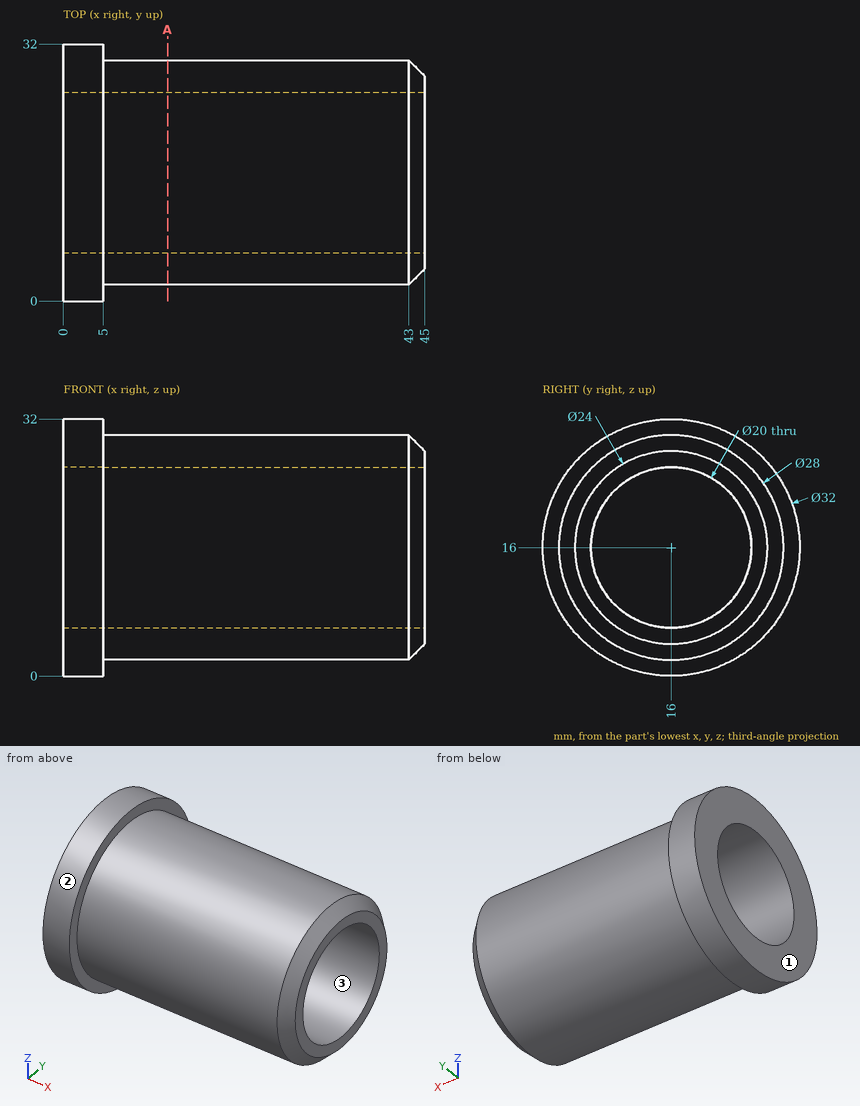
Could you check a few things on this drawing? It's one solid part, dimensions in mm from its lowest x, y, z. Give positions to 0.01 mm unless a question says otherwise; leave off trailing zeros. Order: outer loops, then holes, each group sorted by start corner. A loop starts at its lowest first (then second) coordinate and runs counter-clockwise, first axis right, second up. Notation, with made-up numbers: (20, 71.25) - (62, 71.25) arc R37 ccw to (62, 108.25) - close; hole circle Ø11 at (69, 43). An arc over 180 degrees is marked (long way). One line per item, written item: value. Start each with the question number.
1. Imagine slicing it at A-A on x = 13. List the corners of the cut face in (y, z) for me.
2. Thinking about a two-plate mould opening in Z: for the marked faces 1, 2 and 3, which applies, +Z half, -Z half, draft (parallel to the pull), parting line (faces both ways), or undercut?
3. For P1, Ø10, axis at x = 27, z = 20, coming from the +Y side; P2, Ø8, axis at x = 30, y = 6.5, coming from the -Z side; P3, Ø6, axis at x = 35, y = 24, coming from the +Z side; P4, Ø3, axis at y = 17, z = 24, coming from the +X side, each with a flat end and sliding along its axis, tell me the tip position at first contact or that it passes through.
4. If I drill on probe 1 along Z at (x, y) = (24, 16); probe 2 along Y at (x, z) = (27.5, 17.5); probe 3 along Y at (x, z) = (6, 17), over which ranges is the centre line in solid material (lowest first)?
Values:
1. outline: circle Ø28 at (16, 16); hole circle Ø20 at (16, 16)
2. face 1: draft
2. face 2: parting line
2. face 3: undercut
3. P1: y = 30
3. P2: z = 3.13
3. P3: z = 29.08
3. P4: through
4. probe 1: 2 to 6, 26 to 30
4. probe 2: 2.08 to 6.11, 25.89 to 29.92
4. probe 3: 2.04 to 6.05, 25.95 to 29.96
